Geometry check sheet. Reference: the model listing, model coordinates, mm. Face numbers are marked on the shaded views. A direction names the side the tool comes from. Coordinates: 2 decimals unless noted, no trailing zeros. Loops run counter-clockwise (first coordinate to the right, second up) from the corner with the lowest first, then second, coordinate; pieces in that order, holes last.
from build123d import *


with BuildPart() as part:
    # Sketch1 → Revolve1 (revolve)
    with BuildSketch(Plane.XY):
        with BuildLine():
            Line((0, 0), (0, 1.928074015))
            Line((0, 1.928074015), (57.15, 1.928074015))
            Line((57.15, 1.928074015), (57.15, 36.750137113))
            ThreePointArc((57.15, 36.750137113), (110.052624852, 55.65284987), (162.955249704, 36.750137113))
            ThreePointArc((162.955249704, 36.750137113), (177.8, 5.399105858), (162.955249704, -25.951925396))
            ThreePointArc((162.955249704, -25.951925396), (110.052624852, -44.854638153), (57.15, -25.951925396))
            Line((57.15, -25.951925396), (57.15, -2.834425985))
            Line((57.15, -2.834425985), (0, -2.834425985))
            Line((0, -2.834425985), (0, 0))
        make_face()
    revolve(axis=Axis((0, 0, 0), (0, 1, 0)))


solid = part.part
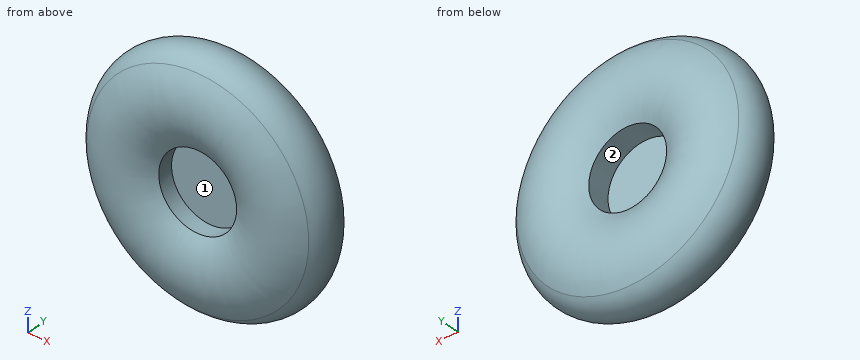
1) Section check D-D on y = -14. Record the cut outline in (x, z).
Data:
outline: circle Ø345.71 at (0, 0); hole circle Ø114.3 at (0, 0)
2) Access from +Z, -Z, +X, -X, +Y, -Y to the whole of each face (thin tool, end or side, straight path). Record for the marked faces 1 and 2.
Data:
face 1: -Y
face 2: +Y
3) Material ranges on probe 1 along Y at (x, z) = (11, -52); probe 2 along X at (y, z) = (-6, -12.5); probe 3 along X at (y, z) = (22, 0), recorded low to high.
Data:
probe 1: y = -2.83 to 1.93
probe 2: x = -175.72 to -55.77, 55.77 to 175.72
probe 3: x = -174.24 to -57.15, 57.15 to 174.24
4) Depth check by flat-ended pin: pin 1 (1 mm diameter, centred on x = -44, y = -23, fed in from +Z); pin 2 (8 mm diameter, centred on x = -38.5, y = 8.5, fed in from -Z); pin 3 (12 mm diameter, centred on y = 7.5, z = 68, fed in from -X). Enter the tip coordinate at first touch or a pass-through.
Data:
pin 1: stops at z = 160.77
pin 2: stops at z = -174.34
pin 3: stops at x = -166.6
5) Section check C-C on y = 12. Record the cut outline in (x, z), and give its area (4 significant figures).
Data:
outline: circle Ø354.52 at (0, 0); hole circle Ø114.3 at (0, 0)
area: 88,450 mm2
6) Section check B-B on x = 0. Record the cut outline in (y, z).
Data:
outline: (-25.95, -162.96) arc R40.53 ccw to (36.75, -162.96) arc R83.48 ccw to (36.75, -57.15) - (1.93, -57.15) - (1.93, 57.15) - (36.75, 57.15) arc R83.48 ccw to (36.75, 162.96) arc R40.53 ccw to (-25.95, 162.96) arc R83.48 ccw to (-25.95, 57.15) - (-2.83, 57.15) - (-2.83, -57.15) - (-25.95, -57.15) arc R83.48 ccw to start
7) Section check A-A on z = 0. Record the cut outline in (x, y), and give its area (3 significant figures).
Data:
outline: (-162.96, -25.95) arc R83.48 ccw to (-57.15, -25.95) - (-57.15, -2.83) - (57.15, -2.83) - (57.15, -25.95) arc R83.48 ccw to (162.96, -25.95) arc R40.53 ccw to (162.96, 36.75) arc R83.48 ccw to (57.15, 36.75) - (57.15, 1.93) - (-57.15, 1.93) - (-57.15, 36.75) arc R83.48 ccw to (-162.96, 36.75) arc R40.53 ccw to start
area: 20,600 mm2
